```python
from build123d import *

# Parameters (mm, degrees)
SKETCH_1_W      = 40
SKETCH_1_H      = 40
EXTRUDE_1_DEPTH = 19
SKETCH_2_R      = 3
EXTRUDE_2_DEPTH = 4
SKETCH_3_W      = 2.45
SKETCH_3_H      = 19
EXTRUDE_3_DEPTH = 7.3
SKETCH_5_W      = 2.45
SKETCH_5_H      = 19
EXTRUDE_4_DEPTH = 7.3


with BuildPart() as part:
    # Эскиз1 → Бобышка-Вытянуть1 (new body)
    with BuildSketch(Plane(origin=(0, 0, 0), x_dir=(1, 0, 0), z_dir=(0, 1, 0))):
        Rectangle(SKETCH_1_W, SKETCH_1_H)
    extrude(amount=EXTRUDE_1_DEPTH)

    # Эскиз2 → Бобышка-Вытянуть2 (add)
    with BuildSketch(Plane(origin=(0, 0, -20), x_dir=(-1, 0, 0), z_dir=(0, 0, -1))):
        with Locations(Location((-11, 10, 0), (0, 0, 180))):
            Circle(SKETCH_2_R)
    extrude(amount=EXTRUDE_2_DEPTH)

    # Эскиз3 → Бобышка-Вытянуть3 (add)
    with BuildSketch(Plane(origin=(20, 0, 0), x_dir=(0, 0, -1), z_dir=(1, 0, 0))):
        with Locations((8.925, 9.5)):
            Rectangle(SKETCH_3_W, SKETCH_3_H)
    extrude(amount=EXTRUDE_3_DEPTH)

    # Эскиз5 → Бобышка-Вытянуть4 (add)
    with BuildSketch(Plane.ZY.offset(20)):
        with Locations((-8.925, 9.5)):
            Rectangle(SKETCH_5_W, SKETCH_5_H)
    extrude(amount=EXTRUDE_4_DEPTH)


solid = part.part
```
Read the model definition and answer for the solid it produces. Units are mm, in the model's axes. A direction names the side the tool comes from. Round coordinates to 2 decimals unless told otherwise and drop trailing zeros. Write each loop counter-clockwise with the first axis right and the second up, starting at its lowest first coordinate (ties: lowest second). Pieces come first, ordered by that corner, then holes. Notation, with made-up numbers: (87.5, 86.5) - (126.5, 86.5) arc R32 ccw to (126.5, 113.5) - close; hole circle Ø4 at (69.5, 60). An arc over 180 degrees is marked (long way). Use CSV: the item, a comma, the result in double quotes.
Q1. Straight lines are drawn through the part: line 1 along Z through (x, y) = (3.5, 14.5); line 2 along Z through (x, y) = (-21.5, 7.25). For each, find the intervals that lie inside material, in ascending order.
Values:
line 1,"z = -20 to 20"
line 2,"z = -10.15 to -7.7"
Q2. Each of these flat-tipped pins is pushed along its axis until it touches: pin 1 Ø2 at (x, y) = (-25, 7) entering from +Z; pin 2 Ø1 at (y, z) = (3.5, -15.5) entering from +X; pin 3 Ø2 at (x, y) = (-22, 10.5) entering from -Z. Where does it stop, or does it pass through?
Values:
pin 1,"stops at z = -7.7"
pin 2,"stops at x = 20"
pin 3,"stops at z = -10.15"
Q3. Find section A-A, the plane y = 6. Write down the section's boundary in (x, z).
Values:
outline,"(-27.3, -10.15) - (-20, -10.15) - (-20, -20) - (20, -20) - (20, -10.15) - (27.3, -10.15) - (27.3, -7.7) - (20, -7.7) - (20, 20) - (-20, 20) - (-20, -7.7) - (-27.3, -7.7) - close"
Q4. Find section D-D, the plane y = 9.25. Write down the section's boundary in (x, z), then the cut area to 3 significant figures.
Values:
outline,"(-27.3, -10.15) - (-20, -10.15) - (-20, -20) - (8.1, -20) - (8.1, -24) - (13.9, -24) - (13.9, -20) - (20, -20) - (20, -10.15) - (27.3, -10.15) - (27.3, -7.7) - (20, -7.7) - (20, 20) - (-20, 20) - (-20, -7.7) - (-27.3, -7.7) - close"
area,"1,660 mm²"
Q5. Find section B-B, the plane x = 11. Write down the section's boundary in (y, z), then the cut area to 3 significant figures.
Values:
outline,"(0, -20) - (7, -20) - (7, -24) - (13, -24) - (13, -20) - (19, -20) - (19, 20) - (0, 20) - close"
area,"784 mm²"
Q6. A tool of negligible diameter and unlimited length cuts with its end or side. For faces 1 (the flat face through (-24, 9, -10.15)), 2 (the flat face through (24, 9, -10.15)), 3 (the flat face through (-20, 9, 6)), 4 (the flat face through (24, 9, -7.7)), 5 (the cylindrical face through (8.79, 7.97, -21.97)), from which of +Z, -Z, +X, -X, +Y, -Y can it reach the whole face along a straight path? Write none if from no direction.
Values:
face 1,"-Z, -X, +Y, -Y"
face 2,"-Z, +X, +Y, -Y"
face 3,"+Z, -X, +Y, -Y"
face 4,"+Z, +X, +Y, -Y"
face 5,"-Z"
Q7. Find section C-C, the plane z = 1.5. Write down the section's boundary in (x, y).
Values:
outline,"(-20, 0) - (20, 0) - (20, 19) - (-20, 19) - close"
